Here's how the part is built. I have some questions about the finished solid (model axes, mm). Give positions to 0.01 mm unless a question says otherwise; leave off trailing zeros. Loops run counter-clockwise (first coordinate to the right, second up) from the corner with the lowest first, then second, coordinate; pieces in that order, holes last.
Q1. Will these pins go through, and if not, where does the flat tip stop? P1, Ø1.5, axis at x = -8.5, z = -39, coming from the +Y side; P2, Ø1.2, axis at y = 6.5, z = -97, coming from the +X side; P3, Ø0.8, axis at x = -10, z = -2.5, coming from the +Y side.
Q2. I need wall thicknesses on line 1 (Y direction, x = -3, z = -91). Which ranges of the line are inside material? Lowest first, please.
Q3. If we section it at C-C (z = -85): Please give me the cut outline in (x, y), plus the area to 3 significant figures.
Q4. If we section it at A-A (z = -2.5): Please give me the cut outline in (x, y).
Q5. If we section it at B-B (x = -5): Please give me the cut outline in (y, z).
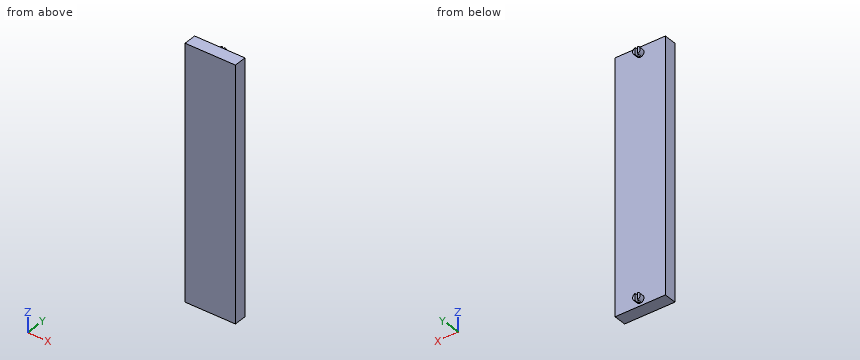
Autodesk Inventor part; units mm, degrees
ref_plane "YZ Plane" through (0, 0, 0) normal (1, 0, 0) x (0, 1, 0)
ref_plane "XZ Plane" through (0, 0, 0) normal (0, 1, 0) x (-1, 0, 0)
ref_plane "XY Plane" through (0, 0, 0) normal (0, 0, 1) x (1, 0, 0)
sketch "Sketch1" plane through (0, 0, 0) normal (0, 1, 0) x (-1, 0, 0)
  line L0 (0, 0) -> (20, 0)
  line L1 (20, 0) -> (20, -100)
  line L2 (20, -100) -> (0, -100)
  line L3 (0, -100) -> (0, 0)
  dimension "d0" = 20
  dimension "d1" = 100
extrude "Extrusion1" add sketch "Sketch1" along normal blind 5
sketch "Sketch2" plane through (0, 5, 0) normal (0, 1, 0) x (1, 0, 0)
  point P0 (0, 0)
sketch "Sketch3" plane through (0, 5, 0) normal (0, 1, 0) x (1, 0, 0)
  point P0 (0, 0)
sketch "Sketch4" plane through (0, 5, 0) normal (0, 1, 0) x (1, 0, 0)
  point P0 (0, 0)
sketch "Sketch5" plane through (0, 5, 0) normal (0, 1, 0) x (1, 0, 0)
  point P0 (0, 0)
sketch "Sketch6" plane through (0, 5, 0) normal (0, 1, 0) x (1, 0, 0)
  circle A0 centre (-10, 2.5) radius 1.5
  point P0 (0, 0)
  dimension "d4" = 3
extrude "Extrusion2" add sketch "Sketch6" along normal blind 2
sketch "Sketch7" plane through (-10, 7, -2.5) normal (0, 1, 0) x (1, 0, 0)
  line L0 (-0.5, 1.5) -> (0.5, 1.5)
  line L1 (0.5, 1.5) -> (0.5, -1.5)
  line L2 (0.5, -1.5) -> (-0.5, -1.5)
  line L3 (-0.5, -1.5) -> (-0.5, 1.5)
  line L4 (-0.5, 1.5) -> (0.5, -1.5) construction
  line L5 (0.5, 1.5) -> (-0.5, -1.5) construction
  point P0 (10, -2.5)
  point P1 (0, 0)
  dimension "d7" = 1
  dimension "d8" = 3
extrude "Extrusion3" cut sketch "Sketch7" against normal blind 1.5
pattern_linear "Rectangular Pattern1" count 2 spacing 95 along (0, 0, -1) of "Extrusion2", "Extrusion3"
properties material "LCP Plastic"
Check sheet entries:
1. P1: stops at y = 5
1. P2: stops at x = -8.5
1. P3: stops at y = 5.5
2. line 1: y = 0 to 5
3. outline: (-20, 0) - (0, 0) - (0, 5) - (-20, 5) - close
3. area: 100 mm2
4. outline: (-20, 0) - (0, 0) - (0, 5) - (-8.5, 5) - (-8.5, 7) - (-9.5, 7) - (-9.5, 5.5) - (-10.5, 5.5) - (-10.5, 7) - (-11.5, 7) - (-11.5, 5) - (-20, 5) - close
5. outline: (0, -100) - (5, -100) - (5, 0) - (0, 0) - close
